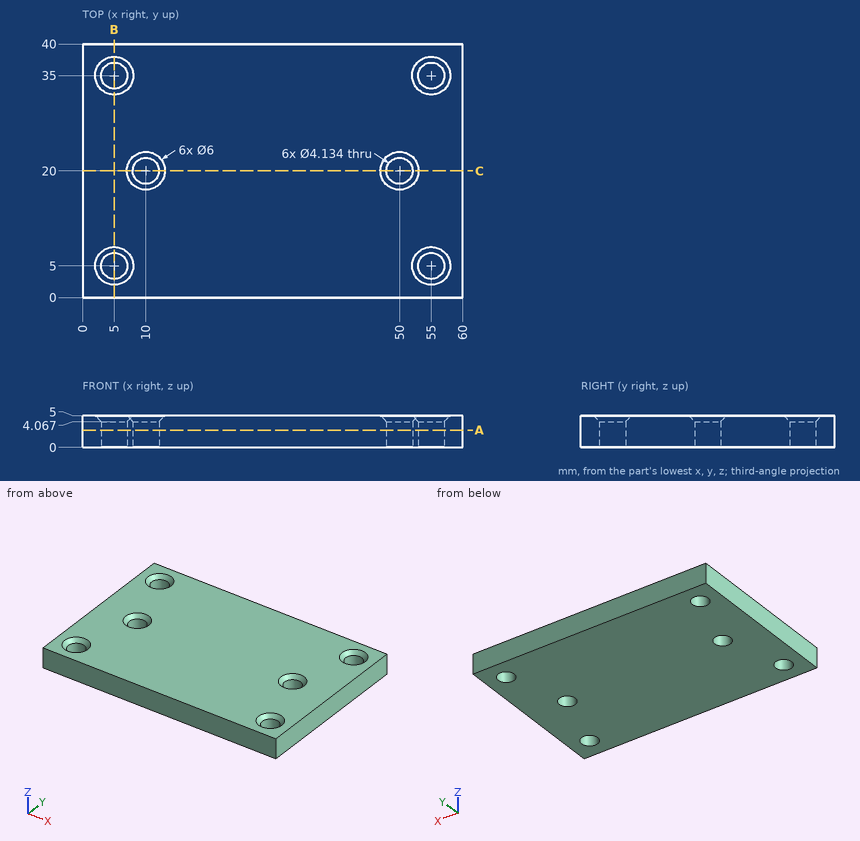
Source: three-view drawing plus pictorial views. Frame: mm from the lowest corner of the part. Round coordinates to 2 decimals unless told otherwise and drop trailing zeros. Write each loop counter-clockwise with the first axis right and the second up, starting at its lowest first coordinate (ties: lowest second). Pieces come first, ordered by that corner, then holes. Notation, with made-up numbers: M 2.25,-20.75 L 21.25,-20.75 A13 ccw 21.25,-0.75 Z; hole C 54.5,48.5 d3. An arc over 180 degrees is marked long. Write each question's results on one line, items separated by ' | '.
Q1. Pin query (flat end, axial travel): P1, Ø2.5, axis at x = 55, y = 5, coming from the +Z side. Return the tip coordinate at first contact, or that it passes through.
Results:
P1: passes through
Q2. Section query A-A (z = 2.7). Return loops of the section in (x, y), and give its area (3 significant figures).
Results:
outline: M 0,0 L 60,0 L 60,40 L 0,40 Z; hole C 5,5 d4.13; hole C 5,35 d4.13; hole C 10,20 d4.13; hole C 50,20 d4.13; hole C 55,5 d4.13; hole C 55,35 d4.13 | area: 2,320 mm^2
Q3. Line query: line 1 along Y through (x, z) = (5, 2.9); line 2 along X through (y, z) = (5, 3.1); line 3 along X through (y, z) = (20, 2.2). Output: solid intervals per line, ascending.
Results:
line 1: y = 0 to 2.93, 7.07 to 32.93, 37.07 to 40 | line 2: x = 0 to 2.93, 7.07 to 52.93, 57.07 to 60 | line 3: x = 0 to 7.93, 12.07 to 47.93, 52.07 to 60
Q4. Section query B-B (x = 5). Return loops of the section in (y, z).
Results:
outline: M 0,0 L 2.93,0 L 2.93,4.07 L 2,5 L 0,5 Z; M 7.07,0 L 32.93,0 L 32.93,4.07 L 32,5 L 8,5 L 7.07,4.07 Z; M 37.07,0 L 40,0 L 40,5 L 38,5 L 37.07,4.07 Z
Q5. Section query C-C (y = 20). Return loops of the section in (x, z), and give its area (3 significant figures).
Results:
outline: M 0,0 L 7.93,0 L 7.93,4.07 L 7,5 L 0,5 Z; M 12.07,0 L 47.93,0 L 47.93,4.07 L 47,5 L 13,5 L 12.07,4.07 Z; M 52.07,0 L 60,0 L 60,5 L 53,5 L 52.07,4.07 Z | area: 257 mm^2
